Check sheet for the modelled part. Datum: model origin and axes. Units: mm. Face numbers are marked on the shaded views. A direction names the side the tool comes from. Round coordinates to 2 decimals unless told otherwise and drop trailing zeros. Order: outer loops, then holes, each group sorted by start corner. A loop starts at its lowest first (then second) coordinate and runs counter-clockwise, first axis right, second up. Notation, with made-up numbers: (-0.75, 50) -> (28.25, 50) arc R35 ccw to (28.25, 82) -> close; hole circle Ø9 at (-16, -21). An arc over 180 degrees is marked (long way). Use CSV: the item, a comma, the result in double quotes.
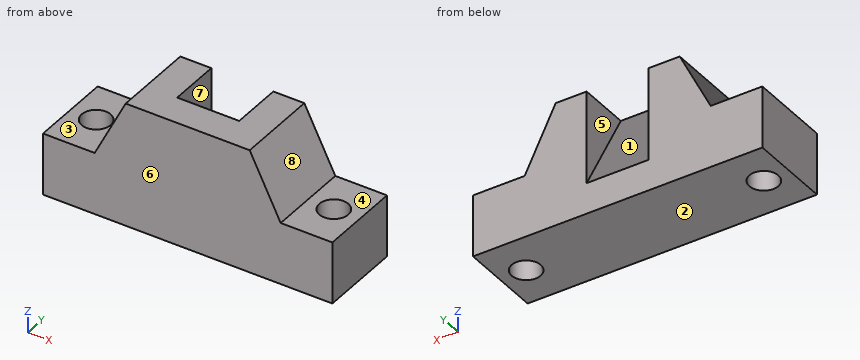
```python
from build123d import *

# Parameters (mm, degrees)
F1_DEPTH      = 40
F2_SIZE2      = 14.99999
F2_SIZE       = 29.99999
F2_2_SIZE2    = 14.99999
F2_2_SIZE     = 29.99999
F3_W          = 30
F3_H          = 45
F4_DEPTH      = 25
F5_SIZE2      = 24.99999
F5_SIZE       = 44.99999
F6_R          = 7
F7_DEPTH      = 15
F7_DEPTH_BACK = 20


# Not quite as in the source:
# - a fillet or chamfer is up to 0.001 mm smaller than in the source, because OpenCascade refuses the exact size


with BuildPart() as f1:
    # F0 (on Front) → F1 (new body)
    with BuildSketch(Plane.XZ):
        Polygon((20.7067526877, 42.941089198), (-69.2932473123, 42.941089198), (-69.2932473123, 12.941089198), (-94.2932473123, 12.941089198), (-94.2932473123, -17.058910802), (45.7067526877, -17.058910802), (45.7067526877, 12.941089198), (20.7067526877, 12.941089198), align=None)
    extrude(amount=F1_DEPTH)

    # F2 (size 30 and 15 in the source; OpenCascade refuses exactly that, so slightly less here)
    f2_edges = [f1.edges().sort_by_distance(p)[0] for p in [
        (-69.293247, -20, 42.941089),
    ]]
    f2_side = f1.faces().sort_by_distance((-69.293247, -20, 27.941089))[0]
    chamfer(f2_edges, length=F2_SIZE, length2=F2_SIZE2, reference=f2_side)

    # F2#2 (size 30 and 15 in the source; OpenCascade refuses exactly that, so slightly less here)
    f2_2_edges = [f1.edges().sort_by_distance(p)[0] for p in [
        (20.706753, -20, 42.941089),
    ]]
    f2_2_side = f1.faces().sort_by_distance((20.706753, -20, 27.941089))[0]
    chamfer(f2_2_edges, length=F2_2_SIZE, length2=F2_2_SIZE2, reference=f2_2_side)

    # F3 (on Front) → F4 (cut)
    with BuildSketch(Plane.XZ):
        with Locations((-24.2932473123, 20.441089198)):
            Rectangle(F3_W, F3_H)
    extrude(amount=F4_DEPTH, mode=Mode.SUBTRACT)

    # F5 (size 45 and 25 in the source; OpenCascade refuses exactly that, so slightly less here)
    f5_edges = [f1.edges().sort_by_distance(p)[0] for p in [
        (-24.293247, -25, -2.058911),
    ]]
    f5_side = f1.faces().sort_by_distance((-24.293247, -25, 20.441089))[0]
    chamfer(f5_edges, length=F5_SIZE, length2=F5_SIZE2, reference=f5_side)

    # F6 (on Top) → F7 (cut, two sides)
    with BuildSketch(Plane.XY) as f7_sk:
        with Locations((-81.7932473123, -20)):
            Circle(F6_R)
        with Locations((33.2067526877, -20)):
            Circle(F6_R)
    extrude(amount=F7_DEPTH, mode=Mode.SUBTRACT)
    extrude(f7_sk.sketch, amount=-F7_DEPTH_BACK, mode=Mode.SUBTRACT)


solid = f1.part
```
Q1. Sectioned sample at B-B, the plane z = 11.5. Enter the section's corners in (x, y), then the cut area to 3 significant figures.
Result sheet:
outline,"(-94.29, -40) -> (45.71, -40) -> (45.71, 0) -> (-9.29, 0) -> (-9.29, -7.53) -> (-39.29, -7.53) -> (-39.29, 0) -> (-94.29, 0) -> close; hole circle Ø14 at (-81.79, -20); hole circle Ø14 at (33.21, -20)"
area,"5,070 mm^2"
Q2. Sectioned sample at C-C, the plane y = -15. State how many separate pieces and enclosed holes the cut face has, then the cut area to 3 significant figures.
Result sheet:
separate pieces,"3"
enclosed holes,"0"
area,"5,320 mm^2"
Q3. Scan lines: L1, parallel to X at y = -20, z = 8.5; L2, parallel to X at y = -22.5, z = 1; L3, parallel to Y at x = 29, z = -6. Record each from-to range of solid material in increasing order.
Result sheet:
L1,"x = -94.29 to -88.79, -74.79 to 26.21, 40.21 to 45.71"
L2,"x = -94.29 to -88.33, -75.25 to 26.67, 39.75 to 45.71"
L3,"y = -40 to -25.59, -14.41 to 0"
Q4. Go/stop test with flat-tipped pins: pin 1 (4 mm diameter, centred on y = -17.5, z = 17.5, fed in from +X); pin 2 (2 mm diameter, centred on x = 20.5, y = -22, fed in from +Z); pin 3 (5 mm diameter, centred on x = -67, y = -16, fed in from +Z). Record where each tip stops, or that it passes through.
Result sheet:
pin 1,"stops at x = 19.43"
pin 2,"stops at z = 15.35"
pin 3,"stops at z = 22.53"
Q5. Mould release check, pull along X, two halves, no side actions. Record for the marked faces 5, 6, 7 and 8: pulls with the +X half, pulls with the -X half, needs draft (parallel to the pull), parting line crosses it, or undercut.
Result sheet:
face 5,"undercut"
face 6,"needs draft"
face 7,"undercut"
face 8,"pulls with the +X half"
Q6. Access from +Z, -Z, +X, -X, +Y, -Y to the whole of each face (thin tool, end or side, straight path). Record for the marked faces 1, 2, 3 and 4.
Result sheet:
face 1,"+Z, +Y"
face 2,"-Z, +X, -X, +Y, -Y"
face 3,"+Z, -X, +Y, -Y"
face 4,"+Z, +X, +Y, -Y"
